Check sheet for the modelled part. Datum: model origin and axes. Units: mm. A direction names the side the tool comes from. Coordinates: 2 decimals unless noted, no trailing zeros. Write each loop counter-clockwise with the first axis right and the second up, starting at its lowest first coordinate (ties: lowest second). Pieces come first, ordered by that corner, then holes. Notation, with made-up numbers: (41, 13) -> (45, 13) arc R25 cw to (45, 40) -> close; hole circle Ø10 at (83, 20). An arc over 180 degrees is marked (long way). One line per item, written item: value. Start each with the question number.
1) Sectioned sample at D-D on x = 4.5. Enter the section's corners in (y, z).
2) Sectioned sample at A-A on x = 0. Enter the section's corners in (y, z).
3) Scan lines: line 1 along Y through (x, z) = (0, 9.75); line 2 along Y through (x, z) = (-4.25, 4). Record each from-to range of solid material in increasing order. Write a range as [from, to].
4) Sectioned sample at B-B on z = 7.5. Enter the section's corners in (x, y), plus the area to 3 significant figures.
5) Set-up check for faces 1 (the cylindrical face through (-1.172, 8.923, 7.395)), 2 (the flat face through (5, -8, 13.2)), 3 (the flat face through (-9.18, -2.46, 14.11)), 4 (the flat face through (2.46, 9.18, 14.11)): record each of +Z, -Z, +X, -X, +Y, -Y from which the full face is reachable in a straight line by a thin tool's end or side.
6) Sectioned sample at C-C on x = -5.5. Enter the section's corners in (y, z).
7) Draft check along Y on faces 5 (the flat face through (-9.4, 0, 13.2)), 6 (the cylindrical face through (-5.75, -5.27, 7.4)), 7 (the flat face through (-9.17, 2.457, 14.113)). Enter one of: +Y half, -Y half, draft (parallel to the pull), parting line (faces both ways), or undercut.
8) Gauge pin test, flat ends, axial feed: P1, Ø2, axis at y = 2.5, z = 4.5, coming from the +X side; P2, Ø5, axis at x = 2.5, y = -3, coming from the +Z side. Record the tip position at first contact, or that the pin passes through.
```python
from build123d import *

# Parameters (mm, degrees)
F0_R     = 9
F1_DEPTH = 15
F3_DEPTH = 1.8
F4_R     = 7.8
F5_DEPTH = 25


with BuildPart() as f1:
    # F0 (on Top) → F1 (new body)
    with BuildSketch(Plane.XY):
        Circle(F0_R)
    extrude(amount=F1_DEPTH)

    # F2 (on face) → F3 (join)
    with BuildSketch(Plane.XY.offset(15)):
        with BuildLine():
            Line((6.363961, 6.363961), (7.071068, 7.071068))
            ThreePointArc((7.071068, 7.071068), (6.087614, 7.933533), (5, 8.660254))
            ThreePointArc((5, 8.660254), (3.826834, 9.238795), (2.58819, 9.659258))
            Line((2.58819, 9.659258), (2.329371, 8.693332))
            ThreePointArc((2.329371, 8.693332), (4.5, 7.794229), (6.363961, 6.363961))
        make_face()
        with BuildLine():
            ThreePointArc((5, -8.660254), (6.087614, -7.933533), (7.071068, -7.071068))
            Line((7.071068, -7.071068), (6.363961, -6.363961))
            ThreePointArc((6.363961, -6.363961), (4.5, -7.794229), (2.329371, -8.693332))
            Line((2.329371, -8.693332), (2.58819, -9.659258))
            ThreePointArc((2.58819, -9.659258), (3.826834, -9.238795), (5, -8.660254))
        make_face()
        with BuildLine():
            Line((-8.693332, 2.329371), (-9.659258, 2.58819))
            ThreePointArc((-9.659258, 2.58819), (-9.914449, 1.305262), (-10, 0))
            ThreePointArc((-10, 0), (-9.914449, -1.305262), (-9.659258, -2.58819))
            Line((-9.659258, -2.58819), (-8.693332, -2.329371))
            ThreePointArc((-8.693332, -2.329371), (-9, 0), (-8.693332, 2.329371))
        make_face()
    extrude(amount=-F3_DEPTH)

    # F4 (on face) → F5 (cut)
    with BuildSketch(Plane(origin=(0, 0, 0), x_dir=(1, 0, 0), z_dir=(0, 0, -1))):
        Circle(F4_R)
    extrude(amount=-F5_DEPTH, mode=Mode.SUBTRACT)


solid = f1.part
```
Answers:
1. outline: (-8.93, 13.2) -> (-7.79, 13.2) -> (-7.79, 0) -> (-6.37, 0) -> (-6.37, 15) -> (-8.93, 15) -> close; (6.37, 0) -> (7.79, 0) -> (7.79, 13.2) -> (8.93, 13.2) -> (8.93, 15) -> (6.37, 15) -> close
2. outline: (-9, 0) -> (-7.8, 0) -> (-7.8, 15) -> (-9, 15) -> close; (7.8, 0) -> (9, 0) -> (9, 15) -> (7.8, 15) -> close
3. line 1: y = [-9, -7.8], [7.8, 9]
3. line 2: y = [-7.93, -6.54], [6.54, 7.93]
4. outline: circle Ø18 at (0, 0); hole circle Ø15.6 at (0, 0)
4. area: 63.3 mm2
5. face 1: -Z
5. face 2: -Z, +X, -Y
5. face 3: +Z, -Z, -Y
5. face 4: +Z, -Z, +Y
6. outline: (-7.12, 0) -> (-5.53, 0) -> (-5.53, 15) -> (-7.12, 15) -> close; (5.53, 0) -> (7.12, 0) -> (7.12, 15) -> (5.53, 15) -> close
7. face 5: draft
7. face 6: undercut
7. face 7: +Y half
8. P1: stops at x = 8.87
8. P2: passes through
